CAD build for the part. Positions are in the model's coordinates, mm. A direction names the side the tool comes from. Round coordinates to 2 decimals unless told otherwise and drop trailing zeros. Loops run counter-clockwise (first coordinate to the right, second up) from the corner with the lowest first, then second, coordinate; pieces in that order, holes last.
from build123d import *

# Parameters (mm, degrees)
SKETCH1_R           = 32
SKETCH1_R_2         = 15
BOSS_EXTRUDE1_DEPTH = 10
SKETCH2_R           = 19
SKETCH2_R_2         = 15
BOSS_EXTRUDE2_DEPTH = 10
SKETCH6_R           = 4
CUT_EXTRUDE1_DEPTH  = 11


with BuildPart() as part:
    # Sketch1 → Boss-Extrude1 (new body)
    with BuildSketch(Plane.XY):
        Circle(SKETCH1_R)
        Circle(SKETCH1_R_2, mode=Mode.SUBTRACT)
    extrude(amount=BOSS_EXTRUDE1_DEPTH)

    # Sketch2 → Boss-Extrude2 (add)
    with BuildSketch(Plane.XY.offset(10)):
        Circle(SKETCH2_R)
        Circle(SKETCH2_R_2, mode=Mode.SUBTRACT)
    extrude(amount=BOSS_EXTRUDE2_DEPTH)

    # Sketch6 → Cut-Extrude1 (cut, through all)
    with BuildSketch(Plane.XY.offset(10)):
        with Locations((-21.650635095, 12.5)):
            Circle(SKETCH6_R)
        with Locations((0, 25)):
            Circle(SKETCH6_R)
        with Locations((21.650635095, 12.5)):
            Circle(SKETCH6_R)
        with Locations((21.650635095, -12.5)):
            Circle(SKETCH6_R)
        with Locations((0, -25)):
            Circle(SKETCH6_R)
        with Locations((-21.650635095, -12.5)):
            Circle(SKETCH6_R)
    extrude(amount=-CUT_EXTRUDE1_DEPTH, mode=Mode.SUBTRACT)


solid = part.part
Item 1: 3-axis set-ups, long thin cutter, end or side, ignore diameter. For faces 4 (the cylindrical face through (25.466, 13.701, 5.07)), 5 (the flat face through (14, -14, 10)): which of +Z, -Z, +X, -X, +Y, -Y reach the whole face in a straight line?
Verdict:
face 4: +Z, -Z
face 5: +Z
Item 2: Cut at B-B (x = 0). List the corners of the cut face in (y, z).
Verdict:
outline: (-32, 0) - (-29, 0) - (-29, 10) - (-32, 10) - close; (-21, 0) - (-15, 0) - (-15, 20) - (-19, 20) - (-19, 10) - (-21, 10) - close; (15, 0) - (21, 0) - (21, 10) - (19, 10) - (19, 20) - (15, 20) - close; (29, 0) - (32, 0) - (32, 10) - (29, 10) - close
Item 3: Flat gauge pins, fed straight in: P1, Ø5, axis at y = 3.5, z = 14, coming from the -X side; P2, Ø10, axis at y = -17, z = 13, coming from the +X side; P3, Ø12, axis at x = -24, z = 12.5, coming from the -Y side. Where does each tip first touch, or does it go through?
Verdict:
P1: stops at x = -18.97
P2: stops at x = 29.24
P3: stops at y = -26.08
Item 4: Mould opens along X. For faces 1 (the cylindrical face through (-6.94, -31.24, 4.93)), 2 (the cylindrical face through (-14.985, 0.66, 9.86)), 3 (the flat face through (7, -14, 0)) say: released by +X, released by -X, zero draft, split by the parting line, or undercut.
Verdict:
face 1: split by the parting line
face 2: undercut
face 3: zero draft
Item 5: Cut at D-D (x = 8). List the corners of the cut face in (y, z), plus the area to 3 significant figures.
Verdict:
outline: (-30.98, 0) - (-12.69, 0) - (-12.69, 20) - (-17.23, 20) - (-17.23, 10) - (-30.98, 10) - close; (12.69, 0) - (30.98, 0) - (30.98, 10) - (17.23, 10) - (17.23, 20) - (12.69, 20) - close
area: 457 mm2
Item 6: Cut at A-A (y = 0). List the corners of the cut face in (x, z), plus the area to 3 significant figures.
Verdict:
outline: (-32, 0) - (-15, 0) - (-15, 20) - (-19, 20) - (-19, 10) - (-32, 10) - close; (15, 0) - (32, 0) - (32, 10) - (19, 10) - (19, 20) - (15, 20) - close
area: 420 mm2
Item 7: Wall check: L1, parallel to Y at x = 0, z = 6.5; L2, parallel to Z at x = -26, y = 10; L3, parallel to X at y = 17, z = 14.5. Give the ranges that are in metal, low to high.
Verdict:
L1: y = -32 to -29, -21 to -15, 15 to 21, 29 to 32
L2: z = 0 to 10
L3: x = -8.49 to 8.49
Item 8: Cut at C-C (z = 9.25). List the corners of the cut face in (x, y).
Verdict:
outline: circle Ø64 at (0, 0); hole circle Ø8 at (-21.65, -12.5); hole circle Ø8 at (-21.65, 12.5); hole circle Ø30 at (0, 0); hole circle Ø8 at (0, -25); hole circle Ø8 at (0, 25); hole circle Ø8 at (21.65, -12.5); hole circle Ø8 at (21.65, 12.5)
